Can you work these out from the model? Positions are in its coordinate system, mm. A direction names the side the tool comes from. Give positions to 0.01 mm unless a question says otherwise; leave off trailing zeros. Loops run counter-clockwise (first coordinate to the right, second up) from the corner with the lowest first, then second, coordinate; pieces in that order, holes last. Notation, with made-up numbers: M -28,64.25 L -4,64.25 A11 ccw -4,81.25 Z; hole C 28,-12 d2. An arc over 180 degrees is marked long. One line per item, written item: value. Start each with the question number.
from build123d import *

# Parameters (mm, degrees)
SKETCH1_R           = 1.5
BOSS_EXTRUDE1_DEPTH = 3


with BuildPart() as part:
    # Sketch1 → Boss-Extrude1 (new body)
    with BuildSketch(Plane(origin=(0, 0, 0), x_dir=(1, 0, 0), z_dir=(0, 1, 0))):
        Polygon((0, 73), (-8.898516379, 68.4375), (-10.267266379, 71.107054914), (-19.165782758, 66.544554914), (-17.797032758, 63.875), (-38.708546249, 53.153125), (-37.294171249, 50.394584922), (-36.13736412, 50.987709922), (-34.99673912, 48.763080828), (-36.153546249, 48.169955828), (-34.419796249, 44.788519604), (-37.089351163, 43.419769604), (-38.823101163, 46.801205828), (-39.979908292, 46.208080828), (-41.120533292, 48.432709922), (-39.963726163, 49.025834922), (-41.378101163, 51.784375), (-62.289614654, 41.0625), (-63.658364654, 43.732054914), (-72.556881033, 39.169554914), (-71.188131033, 36.5), (-92.099644524, 25.778125), (-90.685269524, 23.019584922), (-89.528462395, 23.612709922), (-88.387837395, 21.388080828), (-89.544644524, 20.794955828), (-87.810894524, 17.413519604), (-90.480449438, 16.044769604), (-92.214199438, 19.426205828), (-93.371006567, 18.833080828), (-94.511631567, 21.057709922), (-93.354824438, 21.650834922), (-94.769199438, 24.409375), (-115.680712929, 13.6875), (-117.049462929, 16.357054914), (-125.947979308, 11.794554914), (-124.579229308, 9.125), (-142.376262066, 0), (-128.476262066, 0), (-128.476262066, -3), (-118.476262066, -3), (-118.476262066, 0), (-101.5, 0), (-101.5, 3.1), (-102.8, 3.1), (-102.8, 5.6), (-101.5, 5.6), (-101.5, 9.4), (-98.5, 9.4), (-98.5, 5.6), (-97.2, 5.6), (-97.2, 3.1), (-98.5, 3.1), (-98.5, 0), (-80, 0), (-80, -3), (-70, -3), (-70, 0), (-51.5, 0), (-51.5, 3.1), (-52.8, 3.1), (-52.8, 5.6), (-51.5, 5.6), (-51.5, 9.4), (-48.5, 9.4), (-48.5, 5.6), (-47.2, 5.6), (-47.2, 3.1), (-48.5, 3.1), (-48.5, 0), (-30, 0), (-30, -3), (-20, -3), (-20, 0), (0, 0), (0, 15), (3, 15), (3, 25), (0, 25), (0, 35), (-3.1, 35), (-3.1, 33.7), (-5.6, 33.7), (-5.6, 35), (-9.4, 35), (-9.4, 38), (-5.6, 38), (-5.6, 39.3), (-3.1, 39.3), (-3.1, 38), (0, 38), (0, 48), (3, 48), (3, 58), (0, 58), align=None)
        with Locations(Location((-27.355510267, 38.424597543, 0), (0, 0, 270))):
            Circle(SKETCH1_R, mode=Mode.SUBTRACT)
        Polygon((-18.2, 44.675), (-23.094184009, 42.165625), (-21.725434009, 39.496070086), (-16.83125, 42.005445086), align=None, mode=Mode.SUBTRACT)
        Polygon((-32.858434402, 37.159240731), (-31.489684402, 34.489685817), (-36.383868411, 31.980310817), (-37.752618411, 34.649865731), align=None, mode=Mode.SUBTRACT)
        with BuildLine():
            Line((-48.5, 33.56496631), (-48.5, 25.598461138))
            Line((-48.5, 25.598461138), (-51.491944896, 25.598461138))
            Line((-51.491944896, 25.598461138), (-51.491944896, 32.995360227))
            ThreePointArc((-51.491944896, 32.995360227), (-56.315394441, 28.171910682), (-51.491944896, 23.348461138))
            Line((-51.491944896, 23.348461138), (-48.5, 23.348461138))
            Line((-48.5, 23.348461138), (-48.5, 21.548461138))
            ThreePointArc((-48.5, 21.548461138), (-59.151745227, 29.1370418), (-48.5, 36.725622462))
            ThreePointArc((-48.5, 36.725622462), (-47.33660311, 37.110417568), (-46.55, 38.05))
            ThreePointArc((-46.55, 38.05), (-46.596119109, 35.403624932), (-48.5, 33.56496631))
        make_face(mode=Mode.SUBTRACT)
        with BuildLine():
            Line((-62.945288743, 22.499922927), (-61.814756339, 21.369390522))
            ThreePointArc((-61.814756339, 21.369390522), (-60.26196681, 23.207262023), (-57.875304833, 22.902677745))
            Line((-57.875304833, 22.902677745), (-59.34866377, 24.848461138))
            ThreePointArc((-59.34866377, 24.848461138), (-61.658382233, 24.457375162), (-62.945288743, 22.499922927))
        make_face(mode=Mode.SUBTRACT)
        with BuildLine():
            Line((-56.219305992, 21.108017954), (-54.281025882, 20.251876901))
            ThreePointArc((-54.281025882, 20.251876901), (-56.459608889, 17.845467185), (-59.295560451, 16.26609694))
            ThreePointArc((-59.295560451, 16.26609694), (-59.670500049, 12.923855807), (-56.562556798, 14.209096735))
            Line((-56.562556798, 14.209096735), (-56.075146683, 13.110422752))
            ThreePointArc((-56.075146683, 13.110422752), (-62.116171263, 12.397132702), (-59.571948462, 17.922500654))
            ThreePointArc((-59.571948462, 17.922500654), (-57.634172668, 19.240087777), (-56.219305992, 21.108017954))
        make_face(mode=Mode.SUBTRACT)
    extrude(amount=BOSS_EXTRUDE1_DEPTH)


solid = part.part
Q1. Which directions (+Z, -Z, +X, -X, +Y, -Y) give clear straight access to the entire face, cutting with the end or side of a thin tool? Please do faces 1 (the face through (-20.61, 1.48, -43.44)), 2 (the face through (-9.4, 1, -36)), 3 (the face through (-40.661, 1.479, -50.386)).
Q2. If we mould it in two halves opening along X, with no side actions, what happens to faces 4 (the face through (-68.05, 1.48, -41.48)), 5 (the face through (-17.506, 1.479, -43.322)), 6 (the face through (-136, 1, 0))? For each: released by +X, released by -X, zero draft, split by the parting line, or undercut.
Q3. For P1, Ø1, axis at x = -95, y = 1.5, coming from the +Z side; P2, Ø1.5, axis at y = 1, z = 2, coming from the -X side; P3, Ø1.5, axis at x = 1, y = 1.5, coming from the -Z side, each with a flat end and sliding along its axis, tell me the tip position at first contact or that it passes through.
Q4. If we section it at B-B, the plane y = 1.7: Give the number of separate pieces and of enclosed holes in the cut face, plus the area to 3 significant figures.
Q5. I need wall thicknesses on line 1 along X through (y, z) = (2.65, -43); line 2 along Z through (x, y) = (-37, 2.85); line 3 along Z through (x, y) = (-49, 2.1). Which ranges of each line are inside material? Lowest first, please.
Q6. If we section it at A-A, the plane x = -109.5: Write out the boundary of the cut face in (y, z).
Response:
1. face 1: +Y, -Y
1. face 2: +X, +Y, -Y
1. face 3: -Z, +Y, -Y
2. face 4: released by -X
2. face 5: undercut
2. face 6: zero draft
3. P1: z = 0
3. P2: x = -128.48
3. P3: z = -58
4. separate pieces: 1
4. enclosed holes: 6
4. area: 5,080 mm^2
5. line 1: -65.09 to -63.28, -58.51 to -21.47, -17.34 to 0
5. line 2: -54.03 to -50.55, -43.47 to -35.04, -33.18 to 0
5. line 3: -47.88 to -36.88, -25.6 to -23.35, -21.39 to -9.4
6. outline: M 0,-16.86 L 3,-16.86 L 3,0 L 0,0 Z
